For this review, take the finished solid that the model builds, in its own axes (mm). A direction names the side the tool comes from. Give positions to 0.01 mm unless a question says otherwise; leave off trailing zeros. Order: outer loops, then holes, each group sorted by start corner. A loop starts at its lowest first (then second) coordinate and runs counter-clockwise, first axis right, second up. Notation, with made-up numbers: M 10,46.25 L 31,46.25 A22 cw 31,71.25 Z; hole C 17.5,-24.75 d3. An arc over 180 degrees is marked long. Use CSV: the item, a comma, the result in double quotes. Start each with the question number.
(1) Tool access review of faces 5 (the face through (34, 0, 13.6)), 6 (the face through (33.5, 0.1, 8)), 7 (the face through (34.5, 0.1, 8)): name each direction out of +Z, -Z, +X, -X, +Y, -Y from which nothing blocks a thin tool from reaching the whole face with its end or side.
(2) Draft analysis for pull direction X (two halves, no side actions). For faces 1 (the face through (-10, 0, 1)), 2 (the face through (0, 0, 1.6)), 3 (the face through (41, 0, 1.6)), 4 (the face through (45.407, 1.464, 0.811)), state which applies: pulls with the +X half, pulls with the -X half, needs draft (parallel to the pull), parting line crosses it, or undercut.
(3) Wall thickness on L1, parallel to X at y = 0, z = 11; L2, parallel to Y at x = 0, z = 5.5; L3, parallel to X at y = 1, z = 9.75: over which ranges is each line inside the solid? List them lowest first. Write a range as from..to.
(4) Consider section B-B (z = 1). Write out the cut boundary in (x, y).
(5) Clearance check with flat-ended pins moving along their axes: P1, Ø1, axis at x = 28.5, y = -2.5, coming from the +Z side; P2, Ø4.5, axis at x = 0, y = 0, coming from the -Z side; P3, Ø1, axis at y = -2, z = 10, coming from the -X side. State where each tip first meets the part, or that it passes through.
(6) Consider section A-A (z = 9.75). Write out the cut boundary in (x, y), and give its area (3 significant figures).
(7) Consider section C-C (x = 18). Write out the cut boundary in (y, z).
Autodesk Fusion 360 part; units mm, degrees
sketch "Esquisse1" plane through (0, 0, 0) normal (0, 0, 1) x (1, 0, 0)
  line L0 (-10, 4.5) -> (50, 4.5)
  line L1 (50, 4.5) -> (50, -4.5)
  line L2 (50, -4.5) -> (-10, -4.5)
  line L3 (-10, -4.5) -> (-10, 4.5)
  dimension "d1" = 60
  dimension "d2" = 9
  dimension "d3" = 10
  dimension "d4" = 4.5
extrude "Extrusion1" add sketch "Esquisse1" along normal blind 1.6
sketch "Esquisse2" plane through (0, 0, 1.6) normal (0, 0, 1) x (-1, 0, 0)
  line L0 (10, 4.5) -> (-50, 4.5)
  line L1 (-50, 4.5) -> (-50, -4.5)
  line L2 (-50, -4.5) -> (10, -4.5)
  line L3 (10, -4.5) -> (10, 4.5)
  circle A0 centre (0, 0) radius 3.5
  arc A1 (-33.1964, 4.5) -> (-33.1963, -4.5007) centre (0, 0) ccw
  arc A2 (-34.2053, 4.5) -> (-34.2053, -4.5) centre (0, 0) ccw
  line L4 (-33.1963, -4.5007) -> (-34.2053, -4.5)
  line L5 (-33.1963, -4.5007) -> (-34.2053, -4.5)
  line L6 (-33.1964, 4.5) -> (-34.2053, 4.5)
  circle A3 centre (0, 0) radius 2.8
  dimension "d7" = 7
  dimension "d8" = 33.5
  dimension "d9" = 34.5
  dimension "d10" = 5.6
extrude "Extrusion2" add sketch "Esquisse2" along normal blind 12 contours L0 L2 A1 A2 L4 L5 L6
extrude "Extrusion3" add sketch "Esquisse2" along normal blind 12 contours A0
sketch "Esquisse3" plane through (0, 0, 13.6) normal (0, 0, 1) x (-1, 0, 0)
  circle A0 centre (0, 0) radius 2.8
  circle A1 centre (0, 0) radius 3.5
  line L0 (2.0235, -2.7693) -> (-1.9765, -2.7693)
  line L1 (-1.9765, -2.7693) -> (-1.9765, -2.0693)
  line L2 (-1.9765, -2.0693) -> (2.0235, -2.0693)
  line L3 (2.0235, -2.0693) -> (2.0235, -2.7693)
  dimension "d15" = 4
  dimension "d16" = 0.7
extrude "Extrusion4" add sketch "Esquisse3" against normal blind 12.2 contours A0 L0 L1 L2
sketch "Esquisse4" plane through (0, 0, 1.6) normal (0, 0, 1) x (-1, 0, 0)
  circle A0 centre (-50.5342, 10.9358) radius 10.7703
  circle A1 centre (-50.5342, -10.9358) radius 10.7705
  dimension "d19" = 21.5407
  dimension "d20" = 21.541
  dimension "d21" = 10.9358
  dimension "d22" = 10.9358
  dimension "d23" = 50.5342
  dimension "d24" = 50.5342
extrude "Extrusion5" cut sketch "Esquisse4" against normal blind 2
fillet "Congé1" radius 1 1 edges at (3.2631, -1.2657, 1.6)
fillet "Congé2" radius 1 2 edges at (33.5, 0, 1.6) (34.5, 0, 1.6)
Check result:
1,face 5,"+Z, +X, -X, +Y, -Y"
1,face 6,"+Z"
1,face 7,"+Z, +X"
2,face 1,"pulls with the -X half"
2,face 2,"undercut"
2,face 3,"needs draft"
2,face 4,"pulls with the +X half"
3,L1,"x = -3.5..-2.8, 2.8..3.5, 33.5..34.5"
3,L2,"y = -3.5..-2.8, 2.8..3.5"
3,L3,"x = -3.35..-2.62, 2.62..3.35, 33.49..34.49"
4,outline,"M -10,-4.5 L 41.9,-4.5 A10.77 cw 50,-0.18 L 50,0.18 A10.77 cw 41.9,4.5 L -10,4.5 Z"
5,P1,"stops at z = 1.6"
5,P2,"stops at z = 0"
5,P3,"stops at x = -3.16"
6,outline,"C 0,0 d7; M 33.2,-4.5 L 34.21,-4.5 A34.5 ccw 34.21,4.5 L 33.2,4.5 A33.5 cw Z; hole C 0,0 d5.6"
6,area,"22.9 mm^2"
7,outline,"M -4.5,0 L 4.5,0 L 4.5,1.6 L -4.5,1.6 Z"
